from build123d import *

# Parameters (mm, degrees)
ESQUISSE1_W             = 329
ESQUISSE1_H             = 260
BOSS_EXTRU_1_DEPTH      = 370
ESQUISSE2_W             = 309
ESQUISSE2_H             = 330
ENL_V_MAT_EXTRU_1_DEPTH = 190
ESQUISSE11_W            = 228.480314258
ESQUISSE11_H            = 25.470871893
ENL_V_MAT_EXTRU_9_DEPTH = 50


with BuildPart() as part:
    # Esquisse1 → Boss.-Extru.1 (new body)
    with BuildSketch(Plane.XY):
        with Locations((65.728262625, -82.519920319)):
            Rectangle(ESQUISSE1_W, ESQUISSE1_H)
    extrude(amount=-BOSS_EXTRU_1_DEPTH)

    # Esquisse2 → Enlèv. mat.-Extru.1 (cut)
    with BuildSketch(Plane(origin=(0, 47.480079681, 0), x_dir=(1, 0, 0), z_dir=(0, 1, 0))):
        with Locations((65.728262625, 195)):
            Rectangle(ESQUISSE2_W, ESQUISSE2_H)
    extrude(amount=-ENL_V_MAT_EXTRU_1_DEPTH, mode=Mode.SUBTRACT)

    # Esquisse11 → Enlèv. mat.-Extru.9 (cut)
    with BuildSketch(Plane(origin=(0, -212.519920319, 0), x_dir=(-1, 0, 0), z_dir=(0, -1, 0))):
        with Locations((-73.615667683, 12.735435947)):
            Rectangle(ESQUISSE11_W, ESQUISSE11_H)
    extrude(amount=-ENL_V_MAT_EXTRU_9_DEPTH, mode=Mode.SUBTRACT)


solid = part.part
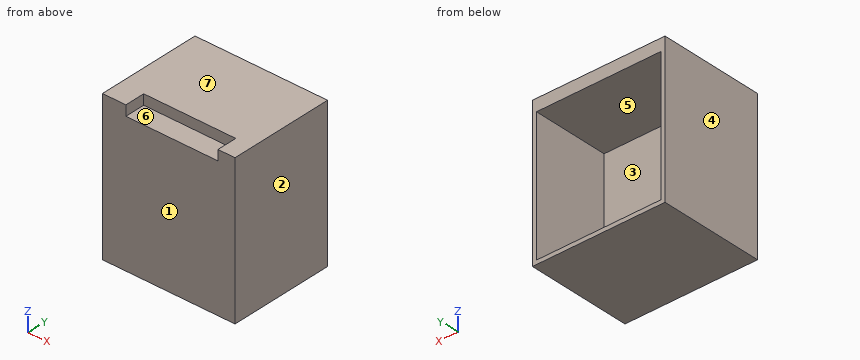
Design review of the part built by this model. Coordinates are the model's own, in mm. Face numbers are marked on the shaded views. A direction names the side the tool comes from. Give positions to 0.01 mm unless a question says otherwise; leave off trailing zeros. Write each loop counter-clockwise with the first axis right and the second up, starting at its lowest first coordinate (ties: lowest second). Pieces come first, ordered by that corner, then holes. Notation, with made-up numbers: M -11.75,-3 L 31.25,-3 A25 cw 31.25,10 Z; hole C 51.5,-12.75 d4. An arc over 180 degrees is marked long. Answer as a JSON object with one key per item and string values. Group by question number.
1) We need section C-C (x = -49.5). Give the boundary of the cut face in (y, z), and give its area (3 significant figures).
2) For line 1 along Z through (x, y) = (67.5, -57); line 2 along X through (y, z) = (-14.5, -110); line 3 along Y through (x, z) = (181, -192.5), list the stretches that pass through material, from the lowest coordinate up.
3) Mouldability with a two-part tool opening along X and no side actions: class the marked faces 1, 2, 3 and 4 as released by +X, released by -X, zero draft, split by the parting line, or undercut.
4) Clearance check with flat-ended pins moving along their axes: pin 1 Ø20.5 at (x, z) = (98.5, -7) entering from -Y; pin 2 Ø15 at (x, y) = (113.5, -194.5) entering from +Z. State where each tip first meets the part, or that it passes through.
5) Tool access review of the marked faces 5, 6 and 7: name each direction out of +Z, -Z, +X, -X, +Y, -Y from which nothing blocks a thin tool from reaching the whole face with its end or side.
6) We need section B-B (z = -39). Give the boundary of the cut face in (x, y).
7) We need section D-D (x = 72). Give the boundary of the cut face in (y, z), and give its area (3 significant figures).
8) We need section A-A (y = -91.5). Give the boundary of the cut face in (x, z).
Answer key:
{
 "1": {"outline": "M -212.52,-370 L 47.48,-370 L 47.48,-360 L -142.52,-360 L -142.52,-30 L 47.48,-30 L 47.48,0 L -212.52,0 Z", "area": "33,500 mm²"},
 "2": {"line 1": "z = -370 to -360, -30 to 0", "line 2": "x = -98.77 to -88.77, 220.23 to 230.23", "line 3": "y = -212.52 to -142.52"},
 "3": {"face 1": "zero draft", "face 2": "released by +X", "face 3": "undercut", "face 4": "released by -X"},
 "4": {"pin 1": "stops at y = -162.52", "pin 2": "stops at z = -25.47"},
 "5": {"face 5": "+Y", "face 6": "+Z, -Y", "face 7": "+Z, +X, -X, +Y, -Y"},
 "6": {"outline": "M -98.77,-212.52 L 230.23,-212.52 L 230.23,47.48 L 220.23,47.48 L 220.23,-142.52 L -88.77,-142.52 L -88.77,47.48 L -98.77,47.48 Z"},
 "7": {"outline": "M -212.52,-370 L 47.48,-370 L 47.48,-360 L -142.52,-360 L -142.52,-30 L 47.48,-30 L 47.48,0 L -162.52,0 L -162.52,-25.47 L -212.52,-25.47 Z", "area": "32,200 mm²"},
 "8": {"outline": "M -98.77,-370 L 230.23,-370 L 230.23,0 L -98.77,0 Z; hole M -88.77,-360 L 220.23,-360 L 220.23,-30 L -88.77,-30 Z"}
}
